from build123d import *

# Parameters (mm, degrees)
SKETCH1_W                        = 38.1
SKETCH1_H                        = 12.7
BOSS_EXTRUDE1_DEPTH              = 50.8
F_1_4_20_TAPPED_HOLE1_AT_2_COUNT = 2
F_1_4_20_TAPPED_HOLE1_AT_2_PITCH = 20.32
F_1_8_0_125_DIAMETER_HOLE1_D     = 3.175
F_1_8_0_125_DIAMETER_HOLE1_DEPTH = 5.08
F_1_8_0_125_DIAMETER_HOLE1_TIP   = 0.953866233


with BuildPart() as part:
    # Sketch1 → Boss-Extrude1 (new body)
    with BuildSketch(Plane.XY):
        Rectangle(SKETCH1_W, SKETCH1_H)
    extrude(amount=-BOSS_EXTRUDE1_DEPTH)

    # Sketch4 → 1/4-20 Tapped Hole1 (revolve, cut)
    with BuildSketch(Plane(origin=(-10.16, 0, 0), x_dir=(0, -1, 0), z_dir=(1, 0, 0))):
        Polygon((0, 0), (0, 14.233816902), (2.5527, 12.7), (2.5527, 0.635), (3.1877, 0), align=None)
    f_1_4_20_tapped_hole1 = revolve(axis=Axis((-10.16, 0, 6.35), (0, 0, -1)), mode=Mode.SUBTRACT)

    # 1/4-20 Tapped Hole1 at 2: 1/4-20 Tapped Hole1 ×2
    with Locations(*[(i * F_1_4_20_TAPPED_HOLE1_AT_2_PITCH, 0, 0) for i in range(1, F_1_4_20_TAPPED_HOLE1_AT_2_COUNT)]):
        add(f_1_4_20_tapped_hole1, mode=Mode.SUBTRACT)

    # Mirror1: 1/4-20 Tapped Hole1 across plane
    add(f_1_4_20_tapped_hole1.mirror(Plane.XY.offset(-25.4)), mode=Mode.SUBTRACT)

    # Mirror1 copy 1 sketch → Mirror1 copy 1 (revolve, cut)
    with BuildSketch(Plane(origin=(10.16, 0, -50.8), x_dir=(0, -1, 0), z_dir=(1, 0, 0))):
        Polygon((0, 0), (0, -14.233816902), (2.5527, -12.7), (2.5527, -0.635), (3.1877, 0), align=None)
    revolve(axis=Axis((10.16, 0, -57.15), (0, 0, -1)), mode=Mode.SUBTRACT)

    # 1/8 (0.125) Diameter Hole1
    with Locations(Plane.ZY.offset(19.05)):
        with Locations((-34.29, 0), (-16.51, 0)):
            Hole(F_1_8_0_125_DIAMETER_HOLE1_D / 2, depth=F_1_8_0_125_DIAMETER_HOLE1_DEPTH)
            with Locations((0, 0, -(F_1_8_0_125_DIAMETER_HOLE1_DEPTH + F_1_8_0_125_DIAMETER_HOLE1_TIP / 2))):  # 118° drill point
                Cone(0, F_1_8_0_125_DIAMETER_HOLE1_D / 2, F_1_8_0_125_DIAMETER_HOLE1_TIP, mode=Mode.SUBTRACT)


solid = part.part
Design review of the part built by this model. Coordinates are the model's own, in mm. A direction names the side the tool comes from. Round coordinates to 2 decimals unless told otherwise and drop trailing zeros. Write each loop counter-clockwise with the first axis right and the second up, starting at its lowest first coordinate (ties: lowest second). Pieces come first, ordered by that corner, then holes. Notation, with made-up numbers: (-13, -30.5) -> (36, -30.5) arc R12 ccw to (36, -23.5) -> close; hole circle Ø2 at (62.25, -37). An arc over 180 degrees is marked (long way). One line per item, written item: value. Start each with the question number.
Q1. Tool access review of faces 5 (the face through (-7.668, 0.553, -6.583)), 6 (the face through (0, 0, 0)), 7 (the face through (-7.668, 0.553, -44.217)), 8 (the face through (-16.474, 0.477, -35.804)): name each direction out of +Z, -Z, +X, -X, +Y, -Y from which nothing blocks a thin tool from reaching the whole face with its end or side.
Q2. Add section B-B (x = -15). State how many separate pieces and enclosed holes the cut face has, then the cut area to 3 significant figures.
Q3. Add section A-A (z = -8.5). Give the boundary of the cut face in (x, y).
Q4. The part is to be moulded in two halves that separate along Y. For faces 1 (the face through (0, -6.35, -25)), 2 (the face through (0, 6.35, -25)), 3 (the face through (0, 0, -50.8)), 4 (the face through (7.63, 0.33, -44.22)), say which applies: pulls with the +Y half, pulls with the -Y half, needs draft (parallel to the pull), parting line crosses it, or undercut.
Q5. Insertion check: P1, Ø6.5, axis at x = 10.16, y = 0, coming from the -Z side; P2, Ø4.5, axis at x = 10.16, y = 0, coming from the +Z side. Each pin has a flat end and moves straight along its axis. Give the tip position at first contact, or say it passes through.
Q6. To check wall thickness, follow probe 1 along X at (y, z) = (0, -45); probe 2 along Z at (x, y) = (-17.35, 0); probe 3 along Y at (x, z) = (-10.16, -43.5). State the ranges of each line that lie inside material, in increasing order.
Response:
1. face 5: +Z
1. face 6: +Z, +X, -X, +Y, -Y
1. face 7: -Z
1. face 8: -X
2. separate pieces: 1
2. enclosed holes: 2
2. area: 629 mm^2
3. outline: (-19.05, -6.35) -> (19.05, -6.35) -> (19.05, 6.35) -> (-19.05, 6.35) -> close; hole circle Ø5.11 at (-10.16, 0); hole circle Ø5.11 at (10.16, 0)
4. face 1: pulls with the -Y half
4. face 2: pulls with the +Y half
4. face 3: needs draft
4. face 4: undercut
5. P1: stops at z = -50.8
5. P2: stops at z = -12.88
6. probe 1: x = -19.05 to -12.71, -7.61 to 7.61, 12.71 to 19.05
6. probe 2: z = -50.8 to -35.88, -32.7 to -18.1, -14.92 to 0
6. probe 3: y = -6.35 to -2.55, 2.55 to 6.35
